Print and shaded views of the part. All mm, measured from the part's lowest x, y and z. A direction names the side the tool comes from. Coordinates: 2 decimals unless noted, no trailing zeros. Loops run counter-clockwise (first coordinate to the right, second up) from the corner with the lowest first, then second, coordinate; pieces in that order, holes last. Notation, with made-up numbers: M 85,5 L 128,5 A32 cw 128,31 Z; hole C 78,64 d8. An arc over 180 degrees is marked long. Use a Markdown table: item, result. Add a question column.
1) Tool access for the marked faces 1 and 2: list every direction of +Z, -Z, +X, -X, +Y, -Y with a clear straight run to the whole face (end or side of a thin tool).
2) Band-saw the part on C-C (x = 2.5). List the corners of the cut face in (y, z).
3) Pull direction Z, two halves, no side cores. Call the marked faces 3, 4 and 5: released by +Z, released by -Z, zero draft, split by the parting line, or undercut.
4) Band-saw the part on A-A (z = 12.5). List the corners of the cut face in (x, y).
5) Pin check, flat tips, straight feed: pin 1 Ø2 at (x, y) = (9.5, 19.5) entering from +Z; pin 2 Ø2 at (x, y) = (1.5, 6) entering from -Z (3 decimals); pin 3 Ø7 at (y, z) = (12.5, 12.5) entering from +X. Stop position of each tip, or through.
6) Wall check: probe 1 along Z at (x, y) = (10.25, 12.5); probe 2 along Z at (x, y) = (7.5, 12.5); probe 3 along Y at (x, z) = (11, 16.25). Give the ranges that are in metal, low to high. Write a range as from..to.
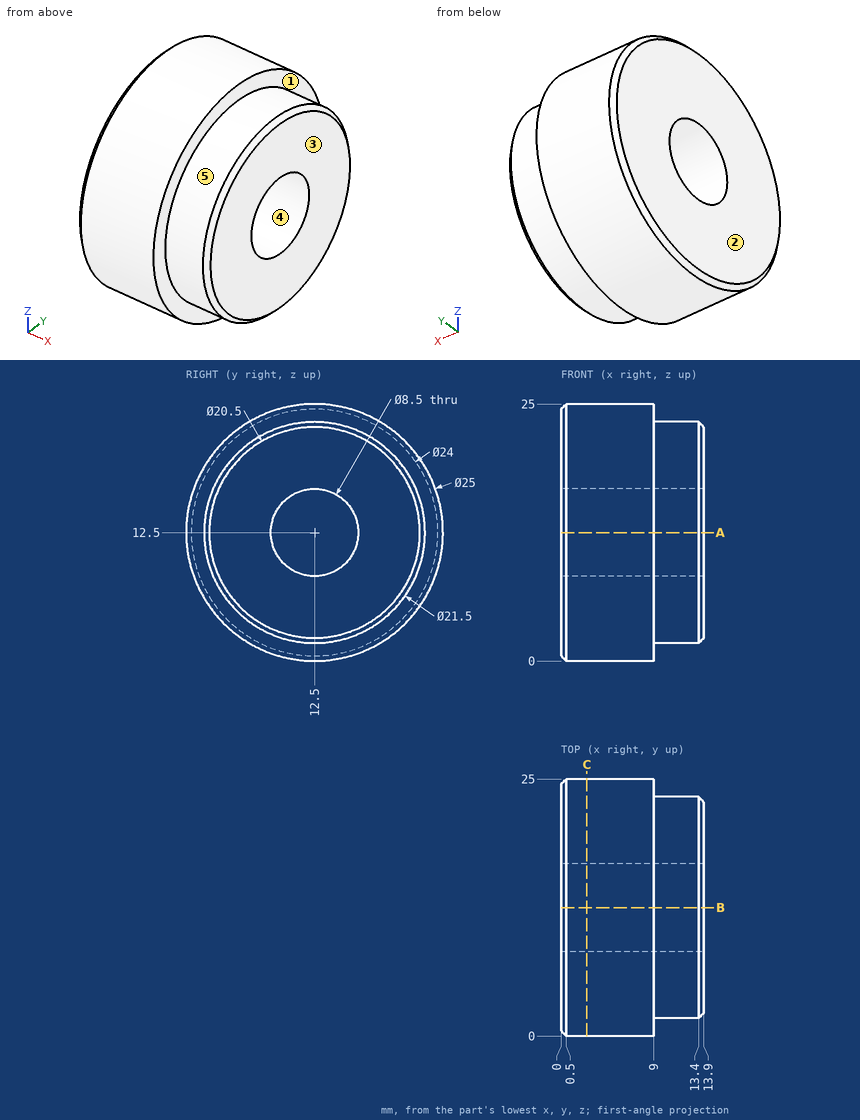
Entries:
| question | item | result |
|---|---|---|
| 1 | face 1 | +X |
| 1 | face 2 | +Z, -Z, -X, +Y, -Y |
| 2 | outline | C 12.5,12.5 d25; hole C 12.5,12.5 d8.5 |
| 3 | face 3 | zero draft |
| 3 | face 4 | undercut |
| 3 | face 5 | split by the parting line |
| 4 | outline | M 0,0.5 L 0.5,0 L 9,0 L 9,1.75 L 13.4,1.75 L 13.9,2.25 L 13.9,8.25 L 0,8.25 Z; M 0,16.75 L 13.9,16.75 L 13.9,22.75 L 13.4,23.25 L 9,23.25 L 9,25 L 0.5,25 L 0,24.5 Z |
| 5 | pin 1 | z = 23.39 |
| 5 | pin 2 | z = 1.275 |
| 5 | pin 3 | through |
| 6 | probe 1 | 1.75..8.25, 16.75..23.25 |
| 6 | probe 2 | 0..8.25, 16.75..25 |
| 6 | probe 3 | 2.43..10.5, 14.5..22.57 |
